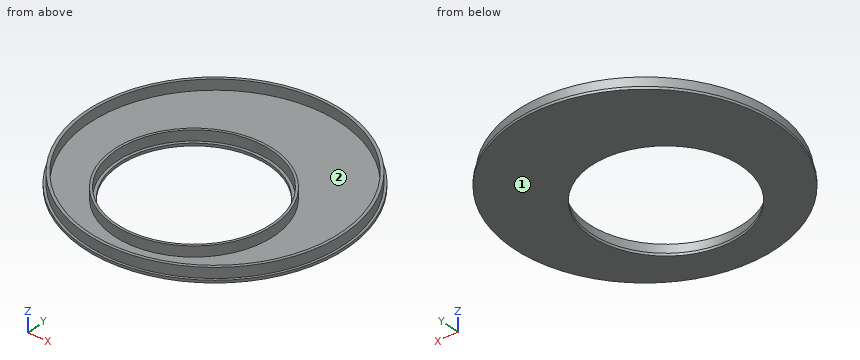
from build123d import *

# Parameters (mm, degrees)
F0_R     = 51
F0_R_2   = 50.1
F1_DEPTH = 1
F0_R_3   = 30.1
F0_R_4   = 29
F0_R_5   = 49
F0_R_6   = 31
F2_DEPTH = 5


with BuildPart() as f1:
    # F0 (on Top) → F1 (new body)
    with BuildSketch(Plane.XY):
        Circle(F0_R)
        Circle(F0_R_2, mode=Mode.SUBTRACT)
    extrude(amount=F1_DEPTH)



with BuildPart() as f1b:
    # F0 (on Top) → F1, piece 2 (new body)
    with BuildSketch(Plane.XY):
        with Locations((0, -10)):
            Circle(F0_R_3)
        with Locations((0, -10)):
            Circle(F0_R_4, mode=Mode.SUBTRACT)
    extrude(amount=F1_DEPTH)


with BuildPart() as f1c:
    # F0 (on Top) → F1, piece 3 (new body)
    with BuildSketch(Plane.XY):
        Circle(F0_R_5)
        with Locations((0, -10)):
            Circle(F0_R_6, mode=Mode.SUBTRACT)
    extrude(amount=F1_DEPTH)


with BuildPart() as f1_1:
    add(f1.part)

    add(f1b.part)  # F2 merges F1b

    add(f1c.part)  # F2 merges F1c
    # F0 (on Top) → F2 (join)
    with BuildSketch(Plane.XY):
        Circle(F0_R_2)
        Circle(F0_R_5, mode=Mode.SUBTRACT)
        with Locations((0, -10)):
            Circle(F0_R_6)
        with Locations((0, -10)):
            Circle(F0_R_3, mode=Mode.SUBTRACT)
    extrude(amount=F2_DEPTH)


solid = f1_1.part
For this review, take the finished solid that the model builds, in its own axes (mm). Face numbers are marked on the shaded views. Round coordinates to 2 decimals unless told otherwise and drop trailing zeros. Write each loop counter-clockwise with the first axis right and the second up, starting at its lowest first coordinate (ties: lowest second). Pieces come first, ordered by that corner, then holes. Notation, with made-up numbers: (5.25, -7) -> (25.25, -7) arc R20 cw to (25.25, 32) -> close; hole circle Ø2 at (86.25, 65). An arc over 180 degrees is marked (long way). Use CSV: the item, a comma, the result in double quotes.
(1) Consider section C-C, the plane z = 1.95. Give the boundary of the cut face in (x, y), plus the area to 3 significant figures.
Computed values:
outline,"circle Ø100.2 at (0, 0); circle Ø62 at (0, -10); hole circle Ø98 at (0, 0); hole circle Ø60.2 at (0, -10)"
area,"515 mm²"
(2) Consider section A-A, the plane x = 0. Give the boundary of the cut face in (y, z).
Computed values:
outline,"(-51, 0) -> (-39, 0) -> (-39, 1) -> (-40.1, 1) -> (-40.1, 5) -> (-41, 5) -> (-41, 1) -> (-49, 1) -> (-49, 5) -> (-50.1, 5) -> (-50.1, 1) -> (-51, 1) -> close; (19, 0) -> (51, 0) -> (51, 1) -> (50.1, 1) -> (50.1, 5) -> (49, 5) -> (49, 1) -> (21, 1) -> (21, 5) -> (20.1, 5) -> (20.1, 1) -> (19, 1) -> close"
(3) To check wall thickness, follow L1, parallel to Y at x = 0, z = 1.8; L2, parallel to X at y = -19, z = 1.2; L3, parallel to Y at x = 21.5, z = 3.55. State the ranges of each line that lie inside material, in increasing order. Write a range as [from, to].
Computed values:
L1,"[-50.1, -49], [-41, -40.1], [20.1, 21], [49, 50.1]"
L2,"[-46.36, -45.17], [-29.66, -28.72], [28.72, 29.66], [45.17, 46.36]"
L3,"[-45.25, -44.03], [-32.33, -31.07], [11.07, 12.33], [44.03, 45.25]"
(4) Consider section D-D, the plane x = 45. Give the boundary of the cut face in (y, z), plus the area to 3 significant figures.
Computed values:
outline,"(-24, 0) -> (24, 0) -> (24, 1) -> (22.02, 1) -> (22.02, 5) -> (19.39, 5) -> (19.39, 1) -> (-19.39, 1) -> (-19.39, 5) -> (-22.02, 5) -> (-22.02, 1) -> (-24, 1) -> close"
area,"69.1 mm²"
(5) Clearance check with flat-ended pins moving along their axes: P1, Ø1, axis at y = -31.5, z = 2.5, coming from the +X side; P2, Ø3, axis at y = 0, z = 4, coming from the -X side; P3, Ø1.5, axis at x = -22.5, z = 2, coming from the -Y side; P4, Ø12, axis at x = 3, y = 7, coming from the -Z side. State where each tip first meets the part, or that it passes through.
Computed values:
P1,"x = 39.36"
P2,"x = -50.1"
P3,"y = -45.13"
P4,"through"
(6) Consider section B-B, the plane y = -24. Give the boundary of the cut face in (x, z), plus the area to 3 significant figures.
Computed values:
outline,"(-45, 0) -> (-25.4, 0) -> (-25.4, 1) -> (-26.65, 1) -> (-26.65, 5) -> (-27.66, 5) -> (-27.66, 1) -> (-42.72, 1) -> (-42.72, 5) -> (-43.98, 5) -> (-43.98, 1) -> (-45, 1) -> close; (25.4, 0) -> (45, 0) -> (45, 1) -> (43.98, 1) -> (43.98, 5) -> (42.72, 5) -> (42.72, 1) -> (27.66, 1) -> (27.66, 5) -> (26.65, 5) -> (26.65, 1) -> (25.4, 1) -> close"
area,"57.4 mm²"
(7) Draft analysis for pull direction X (two halves, no side actions). For the marked faces 1 and 2, state which applies: +X half, -X half, draft (parallel to the pull), parting line (faces both ways), or undercut.
Computed values:
face 1,"draft"
face 2,"undercut"
